from build123d import *

# Parameters (mm, degrees)
BOSS_EXTRUDE1_DEPTH      = 33.5
BOSS_EXTRUDE1_DEPTH_BACK = 33.5
CUT_EXTRUDE1_DEPTH       = 67
CUT_EXTRUDE1_DEPTH_BACK  = 67
SKETCH4_W                = 8
SKETCH4_H                = 32


with BuildPart() as part:
    # Sketch1 → Boss-Extrude1 (new body, two sides)
    with BuildSketch(Plane.XY) as boss_extrude1_sk:
        with BuildLine():
            Line((-38.714708847, 39.285758826), (-23.5, 12))
            ThreePointArc((-23.5, 12), (-24.560660172, 11.560660172), (-25, 10.5))
            Line((-25, 10.5), (-25, 0))
            Line((-25, 0), (25, 0))
            Line((25, 0), (25, 10.5))
            ThreePointArc((25, 10.5), (24.560660172, 11.560660172), (23.5, 12))
            Line((23.5, 12), (0.275280899, 59.640449438))
            ThreePointArc((0.275280899, 59.640449438), (-29.68120414, 69.502386579), (-38.714708847, 39.285758826))
        make_face()
    extrude(amount=BOSS_EXTRUDE1_DEPTH)
    extrude(boss_extrude1_sk.sketch, amount=-BOSS_EXTRUDE1_DEPTH_BACK)

    # Sketch2 → Cut-Extrude1 (cut, two sides)
    with BuildSketch(Plane(origin=(0, 0, 0), x_dir=(0, 0, -1), z_dir=(1, 0, 0))) as cut_extrude1_sk:
        with BuildLine():
            Line((-67, 100), (-67, -1))
            Line((-67, -1), (-33.5, -1))
            Line((-33.5, -1), (-33.5, 10.5))
            ThreePointArc((-33.5, 10.5), (-33.060660172, 11.560660172), (-32, 12))
            Line((-32, 12), (-12, 12))
            ThreePointArc((-12, 12), (-10.939339828, 12.439339828), (-10.5, 13.5))
            Line((-10.5, 13.5), (-10.5, 23))
            Line((-10.5, 23), (-7.5, 23))
            Line((-7.5, 23), (-7.5, 73))
            Line((-7.5, 73), (7.5, 73))
            Line((7.5, 73), (7.5, 23))
            Line((7.5, 23), (10.5, 23))
            Line((10.5, 23), (10.5, 13.5))
            ThreePointArc((10.5, 13.5), (10.939339828, 12.439339828), (12, 12))
            Line((12, 12), (32, 12))
            ThreePointArc((32, 12), (33.060660172, 11.560660172), (33.5, 10.5))
            Line((33.5, 10.5), (33.5, -1))
            Line((33.5, -1), (67, -1))
            Line((67, -1), (67, 100))
            Line((67, 100), (-67, 100))
        make_face()
    extrude(amount=CUT_EXTRUDE1_DEPTH, mode=Mode.SUBTRACT)
    extrude(cut_extrude1_sk.sketch, amount=-CUT_EXTRUDE1_DEPTH_BACK, mode=Mode.SUBTRACT)

    # Sketch3 → Revolve1 (revolve)
    with BuildSketch(Plane(origin=(0, 50, 0), x_dir=(1, 0, 0), z_dir=(0, 1, 0))):
        with BuildLine():
            Line((-19.5, 10.5), (-7.427303532, 10.5))
            ThreePointArc((-7.427303532, 10.5), (-3.5, 0), (-7.427303532, -10.5))
            Line((-7.427303532, -10.5), (-19.5, -10.5))
            Line((-19.5, -10.5), (-19.5, 10.5))
        make_face()
    revolve(axis=Axis((-19.5, 50, 10.5), (0, 0, -1)))

    # Sketch4 → Cut-Revolve1 (revolve, cut)
    with BuildSketch(Plane(origin=(0, 50, 0), x_dir=(1, 0, 0), z_dir=(0, 1, 0))):
        with Locations((-15.5, 0)):
            Rectangle(SKETCH4_W, SKETCH4_H)
    revolve(axis=Axis((-19.5, 50, 16), (0, 0, -1)), mode=Mode.SUBTRACT)

    # Sketch5 → Cut-Revolve2 (revolve, cut)
    with BuildSketch(Plane.XY.offset(26)):
        Polygon((17.5, 13), (24.5, 13), (24.5, 9.5), (22, 9.5), (22, -1), (17.5, -1), align=None)
    revolve(axis=Axis((17.5, -1, 26), (0, 1, 0)), mode=Mode.SUBTRACT)

    # Sketch6 → Cut-Revolve3 (revolve, cut)
    with BuildSketch(Plane.XY.offset(26)):
        Polygon((-17.5, 13), (-10.5, 13), (-10.5, 9.5), (-13, 9.5), (-13, -1), (-17.5, -1), align=None)
    revolve(axis=Axis((-17.5, -1, 26), (0, 1, 0)), mode=Mode.SUBTRACT)

    # Sketch7 → Cut-Revolve4 (revolve, cut)
    with BuildSketch(Plane.XY.offset(-26)):
        Polygon((-17.5, 13), (-10.5, 13), (-10.5, 9.5), (-13, 9.5), (-13, -1), (-17.5, -1), align=None)
    revolve(axis=Axis((-17.5, -1, -26), (0, 1, 0)), mode=Mode.SUBTRACT)

    # Sketch8 → Cut-Revolve5 (revolve, cut)
    with BuildSketch(Plane.XY.offset(-26)):
        Polygon((17.5, 13), (24.5, 13), (24.5, 9.5), (22, 9.5), (22, -1), (17.5, -1), align=None)
    revolve(axis=Axis((17.5, -1, -26), (0, 1, 0)), mode=Mode.SUBTRACT)


solid = part.part
Model file for the job. Use its own axes, mm. A direction names the side the tool comes from. Give positions to 0.01 mm unless a question says otherwise; leave off trailing zeros. Order: outer loops, then holes, each group sorted by start corner. A loop starts at its lowest first (then second) coordinate and runs counter-clockwise, first axis right, second up. Notation, with made-up numbers: (40.5, -17) - (65.5, -17) arc R31 cw to (65.5, 13) - close; hole circle Ø6 at (13, -2). An arc over 180 degrees is marked (long way). Return JSON: item names as keys, results as strings.
1) 3-axis set-ups, long thin cutter, end or side, ignore diameter. For faces 1 (the flat face through (23, 12, 31)), 2 (the flat face through (23, 12, -31)), 3 (the flat face through (-5, 23, -9)), 4 (the flat face through (-18, 9.5, -21)), 5 (the flat face through (-11, 37, -7.5)): which of +Z, -Z, +X, -X, +Y, -Y reach the whole face in a straight line?
Geometry says:
{"face 1": "+Z, +X, -X, +Y", "face 2": "-Z, +X, -X, +Y", "face 3": "-Z, +X, -X", "face 4": "+Y", "face 5": "-Z"}
2) Cut at A-A, the plane z = 3. Give the cut face in (x, y), plus the area to 3 significant figures.
Geometry says:
{"outline": "(-38.71, 39.29) - (-23.5, 12) arc R1.5 ccw to (-25, 10.5) - (-25, 0) - (25, 0) - (25, 10.5) arc R1.5 ccw to (23.5, 12) - (0.28, 59.64) arc R22 ccw (long way) to start; hole circle Ø16 at (-19.5, 50)", "area": "2,990 mm²"}
3) Probe line 1 (Z direction, x = 17.5, y = 10.15); line 2 (X direction, y = 3.5, z = -26); line 3 (Z direction, x = 17.5, y = 6.75). List the from-to ranges inside material, lowest first. Write a range as from..to.
Geometry says:
{"line 1": "-33.5..-33, -19..19, 33..33.5", "line 2": "-25..-22, -13..13, 22..25", "line 3": "-33.5..-30.5, -21.5..21.5, 30.5..33.5"}
4) Flat gauge pins, fed straight in: P1, Ø15.5, axis at x = -14, z = -27, coming from the +Y side; P2, Ø10.5, axis at x = -2.5, y = 18.5, coming from the -Z side; P3, Ø11, axis at x = 17.5, z = -25, coming from the +Y side; P4, Ø5.5, axis at x = 17.5, z = -26, coming from the +Y side. Where does each tip first touch, or does it go through?
Geometry says:
{"P1": "y = 12", "P2": "z = -10.52", "P3": "y = 9.5", "P4": "through"}
5) Cut at B-B, the plane y = 50. Give the cut face in (x, z) (3 decimals), plus the area to 3 significant figures.
Geometry says:
{"outline": "(-41.5, -7.5) - (-33.633, -7.5) arc R16 ccw to (-31.573, -10.5) - (-27.5, -10.5) - (-27.5, 10.5) - (-31.573, 10.5) arc R16 ccw to (-33.633, 7.5) - (-41.5, 7.5) - close; (-11.5, -10.5) - (-7.427, -10.5) arc R16 ccw to (-5.367, -7.5) - (4.975, -7.5) - (4.975, 7.5) - (-5.367, 7.5) arc R16 ccw to (-7.427, 10.5) - (-11.5, 10.5) - close", "area": "519 mm²"}
6) Cut at D-D, the plane x = -17.5. Count the separate pieces of the cut face and the enclosed holes in it, plus the area to 3 significant figures.
Geometry says:
{"separate pieces": "4", "enclosed holes": "0", "area": "1,360 mm²"}
7) Pull direction Y, two halves, no side cores. Call faces 6 (the cylindrical face through (-20.541, 42.068, -0.147)), 7 (the flat face through (-18, 9.5, 31)), 8 (the cylindrical face through (-29.242, 69.725, 0.105)): pulls with the +Y half, pulls with the -Y half, needs draft (parallel to the pull), parting line crosses it, or undercut.
Geometry says:
{"face 6": "undercut", "face 7": "pulls with the +Y half", "face 8": "parting line crosses it"}
8) Cut at C-C, the plane z = 26. Give the cut face in (x, y).
Geometry says:
{"outline": "(-25, 0) - (-22, 0) - (-22, 9.5) - (-24.5, 9.5) - (-24.5, 11.62) arc R1.5 ccw to (-25, 10.5) - close; (-13, 0) - (13, 0) - (13, 9.5) - (10.5, 9.5) - (10.5, 12) - (-10.5, 12) - (-10.5, 9.5) - (-13, 9.5) - close; (22, 0) - (25, 0) - (25, 10.5) arc R1.5 ccw to (24.5, 11.62) - (24.5, 9.5) - (22, 9.5) - close"}
